Design review of the part built by this model. Coordinates are the model's own, in mm. Face numbers are marked on the shaded views. Round coordinates to 2 decimals unless told otherwise and drop trailing zeros. Order: outer loops, then holes, each group sorted by start corner. A loop starts at its lowest first (then second) coordinate and runs counter-clockwise, first axis right, second up. Notation, with made-up numbers: (31, 30.5) - (70, 30.5) arc R28 cw to (70, 55.5) - close; hole circle Ø6 at (6, 49). An arc over 180 degrees is marked (long way). Use CSV: the item, a comma, the result in double quotes.
from build123d import *

# Parameters (mm, degrees)
F3_R     = 25.4
F4_DEPTH = 2.54


# Not quite as in the source:
# - a fillet or chamfer that OpenCascade refuses, or shapes differently, is made with other operations: its cross-section is extruded or revolved along the edge and cut away or added


with BuildPart() as f2:
    # F0 (on Front) → F2 (revolve)
    with BuildSketch(Plane.XZ):
        Polygon((63.5, 13.6071443505), (63.5, 26.3071443505), (38.1, 12.7), (0, 12.7), (0, 0), (38.1, 0), align=None)
    revolve(axis=Axis((0, 0, 37.3074896634), (0, 0, 1)))

    # F3 (on face) → F4 (cut)
    with BuildSketch(Plane.XY.offset(12.7)):
        Circle(F3_R)
    extrude(amount=-F4_DEPTH, mode=Mode.SUBTRACT)

    # F5: fillet of radius 5.08 on 4 edges, made by hand

    # F5_s1 → F5_t2 (revolve)
    with BuildSketch(Plane.XZ):
        with BuildLine():
            ThreePointArc((39.2238860188, 13.3020818618), (38.0616448552, 12.8528190544), (36.8250010386, 12.7))
            Line((36.8250010386, 12.7), (38.1, 12.7))
            Line((38.1, 12.7), (39.2238860188, 13.3020818618))
        make_face()
    revolve(axis=Axis((0, 0, 12.7), (0, 0, 1)))

    # F5_s3 → F5_t4 (revolve)
    with BuildSketch(Plane.XZ):
        with BuildLine():
            ThreePointArc((25.4, 12.7), (23.5405909488, 10.8405909488), (21.0005909488, 10.16))
            Line((21.0005909488, 10.16), (25.4, 10.16))
            Line((25.4, 10.16), (25.4, 12.7))
        make_face()
    revolve(axis=Axis((0, 0, 10.16), (0, 0, 1)))

    # F5_s5 → F5_t6 (revolve, cut)
    with BuildSketch(Plane.XZ):
        with BuildLine():
            ThreePointArc((56.0211150199, 22.3005983857), (61.0296038302, 22.181162535), (63.5, 17.8226802476))
            Line((63.5, 17.8226802476), (63.5, 26.3071443505))
            Line((63.5, 26.3071443505), (56.0211150199, 22.3005983857))
        make_face()
    revolve(axis=Axis((0, 0, 26.3071443505), (0, 0, 1)), mode=Mode.SUBTRACT)

    # F5_s7 → F5_t8 (revolve, cut)
    with BuildSketch(Plane.XZ):
        with BuildLine():
            ThreePointArc((63.5, 16.6487507133), (62.7784822874, 14.0391468831), (60.8188849801, 12.1708325751))
            Line((60.8188849801, 12.1708325751), (63.5, 13.6071443505))
            Line((63.5, 13.6071443505), (63.5, 16.6487507133))
        make_face()
    revolve(axis=Axis((0, 0, 13.6071443505), (0, 0, 1)), mode=Mode.SUBTRACT)


solid = f2.part
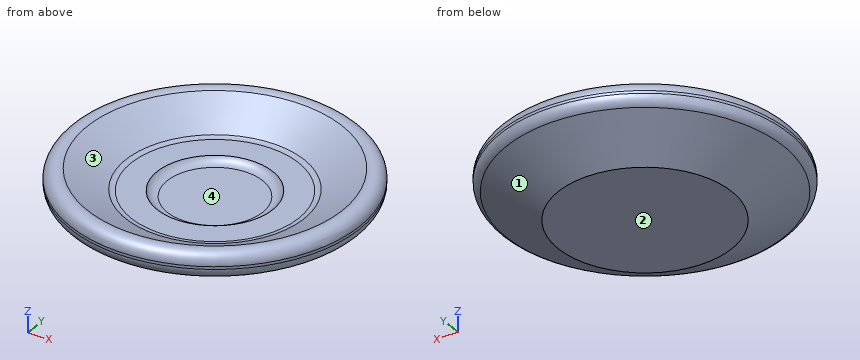
1) To check wall thickness, follow L1, parallel to Y at x = -17, z = 18.75; L2, parallel to Y at x = -30.5, z = 20.75; L3, parallel to Z at x = -26.5, y = -3. State the ranges of each line that lie inside material, in increasing order. Write a range as from..to.
Data:
L1,"y = -61.09..-46.38, 46.38..61.09"
L2,"y = -54.63..-43.5, 43.5..54.63"
L3,"z = 0..12.7"
2) We need section C-C (z = 2). Give the boundary of the cut face in (x, y).
Data:
outline,"circle Ø83.67 at (0, 0)"
3) The part is to be moulded in two halves that separate along Y. For the marked faces 1, 2, 3 and 4, say which applies: +Y half, -Y half, draft (parallel to the pull), parting line (faces both ways), or undercut.
Data:
face 1,"parting line"
face 2,"draft"
face 3,"undercut"
face 4,"undercut"
4) We need section A-A (y = 0). Give the boundary of the cut face in (x, z) (3 decimals), then the cut area to 3 significant figures.
Data:
outline,"(-63.5, 16.649) arc R5.08 ccw to (-60.819, 12.171) - (-38.1, 0) - (38.1, 0) - (60.819, 12.171) arc R5.08 ccw to (63.5, 16.649) - (63.5, 17.823) arc R5.08 ccw to (56.021, 22.301) - (39.224, 13.302) arc R5.08 cw to (36.825, 12.7) - (25.4, 12.7) arc R5.08 cw to (21.001, 10.16) - (-21.001, 10.16) arc R5.08 cw to (-25.4, 12.7) - (-36.825, 12.7) arc R5.08 cw to (-39.224, 13.302) - (-56.021, 22.301) arc R5.08 ccw to (-63.5, 17.823) - close"
area,"1,450 mm2"
5) Insertion check: pin 1 Ø4 at (x, y) = (37.5, 22) entering from -Z; pin 2 Ø12 at (x, y) = (-35.5, -46.5) entering from -Z; pin 3 Ø3 at (x, y) = (12, 35.5) entering from +Z. Each pin has a flat end and moves straight along its axis. Give the tip position at first contact, or say it passes through.
Data:
pin 1,"stops at z = 1.81"
pin 2,"stops at z = 7.72"
pin 3,"stops at z = 13.18"
